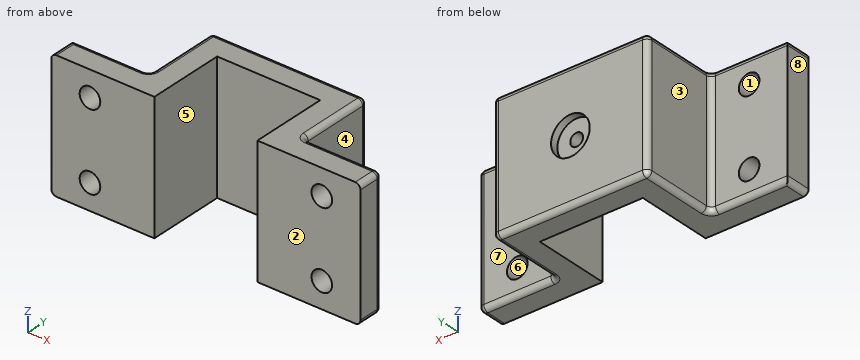
from build123d import *

# Parameters (mm, degrees)
EXTRUDE_THIN1_DEPTH                                 = 31.75
CBORE_FOR_00_BINDING_HEAD_MACHINE_SCREW_D           = 6.35
CBORE_FOR_00_BINDING_HEAD_MACHINE_SCREW_CBORE_D     = 19.05
CBORE_FOR_00_BINDING_HEAD_MACHINE_SCREW_CBORE_DEPTH = 3.81
SKETCH7_R                                           = 5.08
CUT_EXTRUDE1_DEPTH                                  = 91.918163752
LPATTERN1_COUNT                                     = 2
LPATTERN1_PITCH                                     = 38.1
LPATTERN1_COUNT_DIR2                                = 2
LPATTERN1_PITCH_DIR2                                = 114.3
FILLET1_R                                           = 2.54


with BuildPart() as part:
    # Sketch1 → Extrude-Thin1 (new, symmetric)
    with BuildSketch(Plane.XY):
        Polygon((-76.2, 0), (-25.4, 0), (-25.4, 38.1), (25.4, 38.1), (25.4, 0), (76.2, 0), (76.2, 12.7), (38.1, 12.7), (38.1, 50.8), (-38.1, 50.8), (-38.1, 12.7), (-76.2, 12.7), align=None)
    extrude(amount=EXTRUDE_THIN1_DEPTH, both=True)

    # CBORE for #00 Binding Head Machine Screw2 (through all)
    with Locations(Plane(origin=(0, 50.8, 0), x_dir=(1, 0, 0), z_dir=(0, 1, 0))):
        with Locations((0, 0)):
            CounterBoreHole(CBORE_FOR_00_BINDING_HEAD_MACHINE_SCREW_D / 2, CBORE_FOR_00_BINDING_HEAD_MACHINE_SCREW_CBORE_D / 2, CBORE_FOR_00_BINDING_HEAD_MACHINE_SCREW_CBORE_DEPTH)

    # Sketch7 → Cut-Extrude1 (cut, through all)
    with BuildSketch(Plane(origin=(0, 12.7, 0), x_dir=(1, 0, 0), z_dir=(0, 1, 0))):
        with Locations(Location((-57.15, -19.05, 0), (0, 0, 270))):
            Circle(SKETCH7_R)
    cut_extrude1 = extrude(amount=-CUT_EXTRUDE1_DEPTH, mode=Mode.SUBTRACT)

    # LPattern1: Cut-Extrude1 2 × 2
    with Locations(*[(j * LPATTERN1_PITCH_DIR2, 0, -i * LPATTERN1_PITCH) for i in range(LPATTERN1_COUNT) for j in range(LPATTERN1_COUNT_DIR2) if (i, j) != (0, 0)]):
        add(cut_extrude1, mode=Mode.SUBTRACT)

    # Fillet1
    fillet1_edges = [part.edges().sort_by_distance(p)[0] for p in [
        (-76.2, 6.35, -31.75),
        (-57.15, 12.7, -31.75),
        (-38.1, 31.75, -31.75),
        (0, 50.8, -31.75),
        (57.15, 12.7, 31.75),
        (38.1, 31.75, -31.75),
        (57.15, 12.7, -31.75),
        (76.2, 6.35, -31.75),
        (38.1, 31.75, 31.75),
        (-38.1, 12.7, 0),
        (-38.1, 50.8, 0),
        (38.1, 50.8, 0),
        (38.1, 12.7, 0),
        (76.2, 12.7, 0),
        (0, 50.8, 31.75),
        (-38.1, 31.75, 31.75),
        (-57.15, 12.7, 31.75),
        (-76.2, 6.35, 31.75),
        (76.2, 6.35, 31.75),
    ]]
    fillet(fillet1_edges, radius=FILLET1_R)


solid = part.part
Part model, mm, in its own coordinate system. Face numbers are marked on the shaded views. A direction names the side the tool comes from. Coordinates: 2 decimals unless noted, no trailing zeros. Loops run counter-clockwise (first coordinate to the right, second up) from the corner with the lowest first, then second, coordinate; pieces in that order, holes last. Notation, with made-up numbers: M -21,-7 L 32,-7 A19 cw 32,3 Z; hole C -35.75,21.5 d5. An arc over 180 degrees is marked long. Use a Markdown table: item, result. Add a question column.
Q1. Cut at C-C (y = 36). Write the cut outline in (x, z).
Q2. Cut at B-B (z = 19.05). Write the cut outline in (x, y), and give its area (3 significant figures).
Q3. Mould opens along X. For the marked faces 6, 7 and 8 say: +X half, -X half, draft (parallel to the pull), parting line (faces both ways), or undercut.
Q4. Pin check, flat tips, straight feed: P1, Ø25, axis at x = 0, z = 0, coming from the -Y side; P2, Ø11.5, axis at y = 22, z = 4, coming from the +X side; P3, Ø2, axis at y = 45.5, z = 23, coming from the -X side. Stop position of each tip, or through.
Q5. Which spindle directions (+Z, -Z, +X, -X, +Y, -Y) get a long thin tool onto all of the face, cutting with end or side? Do the marked faces 1, 2, 3, 4 and 5. Say none if no direction does.
Q6. Cut at D-D (z = 0). Write the cut outline in (x, y) (3 decimals), and give its area (3 significant figures).
Q7. Cut at A-A (x = 0). Write the cut outline in (y, z) (3 decimals).
Q8. Probe L1, parallel to X at y = 3.75, z = -19.05; L2, parallel to Z at x = -57, y = 3; L3, parallel to X at y = 25, z = 17.5. List the from-to ranges inside material, lowest first.
Worked out:
| question | item | result |
|---|---|---|
| 1 | outline | M -38.1,-29.21 A2.54 ccw -35.56,-31.75 L -25.4,-31.75 L -25.4,31.75 L -35.56,31.75 A2.54 ccw -38.1,29.21 Z; M 25.4,-31.75 L 35.56,-31.75 A2.54 ccw 38.1,-29.21 L 38.1,29.21 A2.54 ccw 35.56,31.75 L 25.4,31.75 Z |
| 2 | outline | M -76.2,0 L -62.23,0 L -62.23,12.7 L -76.2,12.7 Z; M -52.07,0 L -25.4,0 L -25.4,38.1 L 25.4,38.1 L 25.4,0 L 52.07,0 L 52.07,12.7 L 40.64,12.7 A2.54 cw 38.1,15.24 L 38.1,48.26 A2.54 ccw 35.56,50.8 L -35.56,50.8 A2.54 ccw -38.1,48.26 L -38.1,15.24 A2.54 cw -40.64,12.7 L -52.07,12.7 Z; M 62.23,0 L 76.2,0 L 76.2,10.16 A2.54 ccw 73.66,12.7 L 62.23,12.7 Z |
| 2 | area | 2,640 mm2 |
| 3 | face 6 | undercut |
| 3 | face 7 | draft |
| 3 | face 8 | -X half |
| 4 | P1 | stops at y = 38.1 |
| 4 | P2 | stops at x = 38.1 |
| 4 | P3 | stops at x = -38.1 |
| 5 | face 1 | +Y, -Y |
| 5 | face 2 | +Z, -Z, +X, -X, -Y |
| 5 | face 3 | +Z, -Z, -X, +Y |
| 5 | face 4 | +Z, -Z, +X, +Y |
| 5 | face 5 | +Z, -Z, -Y |
| 6 | outline | M -76.2,0 L -25.4,0 L -25.4,38.1 L -3.175,38.1 L -3.175,46.99 L -9.525,46.99 L -9.525,50.8 L -35.56,50.8 A2.54 ccw -38.1,48.26 L -38.1,15.24 A2.54 cw -40.64,12.7 L -76.2,12.7 Z; M 3.175,38.1 L 25.4,38.1 L 25.4,0 L 76.2,0 L 76.2,10.16 A2.54 ccw 73.66,12.7 L 40.64,12.7 A2.54 cw 38.1,15.24 L 38.1,48.26 A2.54 ccw 35.56,50.8 L 9.525,50.8 L 9.525,46.99 L 3.175,46.99 Z |
| 6 | area | 2,770 mm2 |
| 7 | outline | M 38.1,-31.75 L 48.26,-31.75 A2.54 ccw 50.8,-29.21 L 50.8,-9.525 L 46.99,-9.525 L 46.99,-3.175 L 38.1,-3.175 Z; M 38.1,3.175 L 46.99,3.175 L 46.99,9.525 L 50.8,9.525 L 50.8,29.21 A2.54 ccw 48.26,31.75 L 38.1,31.75 Z |
| 8 | L1 | x = -76.2 to -62.23, -52.07 to -25.4, 25.4 to 52.07, 62.23 to 76.2 |
| 8 | L2 | z = -31.75 to -24.13, -13.97 to 13.97, 24.13 to 31.75 |
| 8 | L3 | x = -38.1 to -25.4, 25.4 to 38.1 |
